CAD build for the part. Positions are in the model's coordinates, mm. A direction names the side the tool comes from. Round coordinates to 2 decimals unless told otherwise and drop trailing zeros. Write each loop counter-clockwise with the first axis right and the second up, starting at its lowest first coordinate (ties: lowest second). Pieces come first, ordered by that corner, then holes. Notation, with made-up numbers: (21.5, -29.75) -> (66.5, -29.75) arc R18 ccw to (66.5, -16.75) -> close; hole circle Ø9 at (44.5, 10). An arc over 180 degrees is marked (long way). Answer in a Markdown table with one row per item. Add a question column.
```python
from build123d import *

# Parameters (mm, degrees)
BOSS_EXTRUDE1_START = -71
SKETCH2_W           = 60
SKETCH2_H           = 42
SKETCH2_R           = 7.5
BOSS_EXTRUDE1_DEPTH = 71
SKETCH3_R           = 2.5
SKETCH3_R_2         = 3
SKETCH3_R_3         = 4
CUT_EXTRUDE1_DEPTH  = 97.89169211
SKETCH7_R           = 2.5
CUT_EXTRUDE3_DEPTH  = 81
SKETCH10_R          = 1.25
SKETCH10_R_2        = 0.05
BOSS_EXTRUDE2_DEPTH = 8
CHAMFER10_SIZE      = 1
SKETCH12_R          = 1.5
CUT_EXTRUDE5_DEPTH  = 5
CHAMFER11_SIZE      = 10


with BuildPart() as part:
    # Sketch1 → Revolve1 (revolve)
    with BuildSketch(Plane.XY, mode=Mode.PRIVATE) as revolve1_sk:
        Polygon((0.05, 0), (5, 11.25), (5, 82), (7.5, 82), (7.5, 11.25), (2.55, 0), align=None)
    revolve(revolve1_sk.sketch.rotate(Axis((0, 0, 0), (0, 1, 0)), 90), axis=Axis((0, 0, 0), (0, 1, 0)))

    # Sketch2 → Boss-Extrude1 (add)
    with BuildSketch(Plane(origin=(0, 82, 0), x_dir=(1, 0, 0), z_dir=(0, 1, 0)).offset(BOSS_EXTRUDE1_START)):
        Rectangle(SKETCH2_W, SKETCH2_H)
        with Locations(Location((0, 0, 0), (0, 0, 270))):
            Circle(SKETCH2_R, mode=Mode.SUBTRACT)
    extrude(amount=BOSS_EXTRUDE1_DEPTH)

    # Sketch3 → Cut-Extrude1 (cut, through all)
    with BuildSketch(Plane.XY.offset(21)):
        with Locations((-15, 76)):
            Circle(SKETCH3_R)
        with Locations((-15, 58)):
            Circle(SKETCH3_R_2)
        with Locations((-15, 40)):
            Circle(SKETCH3_R)
        with Locations((15, 76)):
            Circle(SKETCH3_R)
        with Locations((15, 58)):
            Circle(SKETCH3_R_2)
        with Locations((15, 40)):
            Circle(SKETCH3_R)
        with Locations((-8.9, 22.1)):
            Circle(SKETCH3_R_3)
    extrude(amount=-CUT_EXTRUDE1_DEPTH, mode=Mode.SUBTRACT)

    # Sketch7 → Cut-Extrude3 (cut)
    with BuildSketch(Plane(origin=(0, 0, 0), x_dir=(0, 0, 1), z_dir=(-0.9981461553891549, -0.0608625704505587, 0))):
        with Locations(Location((0, 64.5, 0), (0, 0, 270))):
            Circle(SKETCH7_R)
    extrude(amount=-CUT_EXTRUDE3_DEPTH, mode=Mode.SUBTRACT)

    # Sketch10 → Boss-Extrude2 (add)
    with BuildSketch(Plane.XZ):
        with Locations(Location((0, 0, 0), (0, 0, 270))):
            Circle(SKETCH10_R)
        with Locations(Location((0, 0, 0), (0, 0, 90))):
            Circle(SKETCH10_R_2, mode=Mode.SUBTRACT)
    extrude(amount=BOSS_EXTRUDE2_DEPTH)

    # Chamfer10
    chamfer10_edges = [part.edges().sort_by_distance(p)[0] for p in [
        (0, -8, 1.25),
    ]]
    chamfer(chamfer10_edges, length=CHAMFER10_SIZE)

    # Sketch12 → Cut-Extrude5 (cut)
    with BuildSketch(Plane(origin=(0, 82, 0), x_dir=(1, 0, 0), z_dir=(0, 1, 0))):
        with Locations(Location((-15.5, 0, 0), (0, 0, 270))):
            Circle(SKETCH12_R)
        with Locations(Location((-0.1, 15.4, 0), (0, 0, 270))):
            Circle(SKETCH12_R)
        with Locations(Location((15.3, 0, 0), (0, 0, 270))):
            Circle(SKETCH12_R)
        with Locations(Location((0, -15.4, 0), (0, 0, 270))):
            Circle(SKETCH12_R)
    extrude(amount=-CUT_EXTRUDE5_DEPTH, mode=Mode.SUBTRACT)

    # Chamfer11
    chamfer11_edges = [part.edges().sort_by_distance(p)[0] for p in [
        (30, 46.5, -21),
        (30, 46.5, 21),
        (-30, 46.5, 21),
        (-30, 46.5, -21),
    ]]
    chamfer(chamfer11_edges, length=CHAMFER11_SIZE)


solid = part.part
```
Item 1: Saw through at B-B on z = -15.4. Give the cut face in (x, y), then the cut area to 3 significant figures.
Item 2: Saw through at A-A on y = 76. Give the cut face in (x, z), then the cut area to 3 significant figures.
Item 3: Drill centre lines: probe 1 along Y at (x, z) = (15, -7); probe 2 along Y at (x, z) = (-15.5, 11.5); probe 3 along X at (y, z) = (60.5, 2). Where is each one in solid material? Low to high.
Item 4: Pin check, flat tips, straight feed: pin 1 (4 mm diameter, centred on x = -0.1, z = -15.4, fed in from -Y); pin 2 (6 mm diameter, centred on x = 0, z = 9.5, fed in from -Y); pin 3 (3 mm diameter, centred on y = 49, z = 15, fed in from -X). Stop position of each tip, or through.
Item 5: Tool access for faces 1 (the cylindrical face through (-0.03, 79.54, -16.9)), 2 (the flat face through (-25, 46, 16)), 3 (the flat face through (6, 11, -5)): list every direction of +Z, -Z, +X, -X, +Y, -Y with a clear straight run to the whole face (end or side of a thin tool).
Item 6: Saw through at D-D on y = 34. Give the cut face in (x, z), then the cut area to 3 significant figures.
Item 7: Two-plate mould, pull along X, no slides. Class faces 4 (the cylindrical face through (15, 61, 0)), 5 (the flat face through (0, 46, -21)), 6 (the cylindrical face through (-1.22, -3.45, 0.27)): +X half, -X half, draft (parallel to the pull), parting line (faces both ways), or undercut.
Item 8: Saw through at C-C on x = -8.9. Give the cut face in (y, z), then the cut area to 3 significant figures.
Recorded:
| question | item | result |
|---|---|---|
| 1 | outline | (-25.6, 11) -> (25.6, 11) -> (25.6, 82) -> (1.4, 82) -> (1.4, 77) -> (-1.6, 77) -> (-1.6, 82) -> (-25.6, 82) -> close; hole circle Ø6 at (-15, 58); hole circle Ø5 at (-15, 40); hole circle Ø5 at (-15, 76); hole circle Ø8 at (-8.9, 22.1); hole circle Ø6 at (15, 58); hole circle Ø5 at (15, 40); hole circle Ø5 at (15, 76) |
| 1 | area | 3,430 mm2 |
| 2 | outline | (-30, -11) -> (-20, -21) -> (-17.5, -21) -> (-17.5, 21) -> (-20, 21) -> (-30, 11) -> close; (-12.5, -21) -> (12.5, -21) -> (12.5, 21) -> (-12.5, 21) -> close; (17.5, -21) -> (20, -21) -> (30, -11) -> (30, 11) -> (20, 21) -> (17.5, 21) -> close; hole circle Ø10 at (0, 0) |
| 2 | area | 1,820 mm2 |
| 3 | probe 1 | 11 to 37.5, 42.5 to 55, 61 to 73.5, 78.5 to 82 |
| 3 | probe 2 | 11 to 37.55, 42.45 to 55.04, 60.96 to 73.55, 78.45 to 82 |
| 3 | probe 3 | -30 to -16.66, -13.34 to -4.58, 4.58 to 13.34, 16.66 to 30 |
| 4 | pin 1 | y = 11 |
| 4 | pin 2 | y = 8.98 |
| 4 | pin 3 | x = -27.5 |
| 5 | face 1 | +Y |
| 5 | face 2 | +Z, -X, +Y, -Y |
| 5 | face 3 | -Y |
| 6 | outline | (-30, -11) -> (-20, -21) -> (20, -21) -> (30, -11) -> (30, 11) -> (20, 21) -> (-20, 21) -> (-30, 11) -> close; hole circle Ø10 at (0, 0) |
| 6 | area | 2,240 mm2 |
| 7 | face 4 | undercut |
| 7 | face 5 | draft |
| 7 | face 6 | parting line |
| 8 | outline | (11, -21) -> (18.1, -21) -> (18.1, 21) -> (11, 21) -> close; (26.1, -21) -> (82, -21) -> (82, 21) -> (26.1, 21) -> close |
| 8 | area | 2,650 mm2 |
